For this review, use the dimensioned drawing (mm, ordinates from the lowest corner) and the shaded views. A direction names the side the tool comes from. Coordinates: 2 decimals unless noted, no trailing zeros. Write each loop counter-clockwise with the first axis right and the second up, starting at its lowest first coordinate (ties: lowest second). Pieces come first, ordered by that corner, then holes. Notation, with made-up numbers: (85, 3.5) - (93, 3.5) arc R24 ccw to (93, 18.5) - close; hole circle Ø8 at (26, 56). An arc over 180 degrees is marked (long way). One line per item, written item: value.
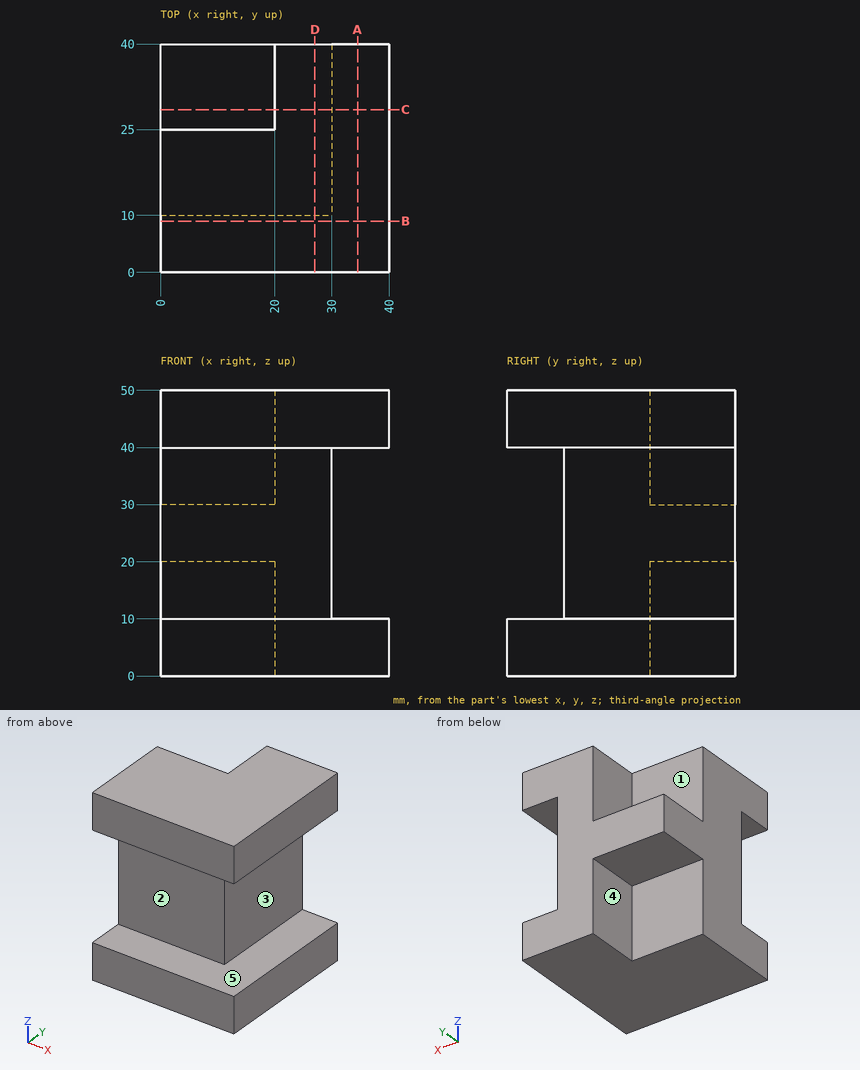
1. Consider section C-C, the plane y = 28.5. Write out the cut boundary in (x, z), then the cut area to 3 significant figures.
Answer block:
outline: (0, 20) - (20, 20) - (20, 0) - (40, 0) - (40, 10) - (30, 10) - (30, 40) - (40, 40) - (40, 50) - (20, 50) - (20, 30) - (0, 30) - close
area: 900 mm^2
2. Wall thickness on line 1 along Z through (x, y) = (19.5, 5.5); line 2 along X through (y, z) = (30, 5); line 3 along Y through (x, z) = (5.5, 24.5): over which ranges is each line inside the solid? List them lowest first.
Answer block:
line 1: z = 0 to 10, 40 to 50
line 2: x = 20 to 40
line 3: y = 10 to 40
3. Consider section A-A, the plane x = 34.5. Write out the cut boundary in (y, z).
Answer block:
outline: (0, 0) - (40, 0) - (40, 10) - (0, 10) - close; (0, 40) - (40, 40) - (40, 50) - (0, 50) - close
4. For the marked faces 1, 2, 3, 4 and 5, list the 3-axis set-ups (+Z, -Z, +X, -X, +Y, -Y) from which the entire face can be reached by the end or side of a thin tool; tool diameter is ignored.
Answer block:
face 1: +Z, -X, +Y
face 2: +X, -X, -Y
face 3: +X, +Y, -Y
face 4: -Z, -X, +Y
face 5: +X, -Y
5. Consider section D-D, the plane x = 27. Write out the cut boundary in (y, z), then the cut area to 3 significant figures.
Answer block:
outline: (0, 0) - (40, 0) - (40, 50) - (0, 50) - (0, 40) - (10, 40) - (10, 10) - (0, 10) - close
area: 1,700 mm^2
6. Insertion check: pin 1 Ø4.5 at (y, z) = (29.5, 43) entering from -X; pin 2 Ø1 at (y, z) = (8, 29.5) entering from -X; pin 3 Ø4 at (x, z) = (4, 26.5) entering from -Y; pin 4 Ø10 at (x, z) = (13.5, 6) entering from +Y. Each pin has a flat end and moves straight along its axis. Give the tip position at first contact, or say it passes through.
Answer block:
pin 1: stops at x = 20
pin 2: passes through
pin 3: stops at y = 10
pin 4: stops at y = 25
